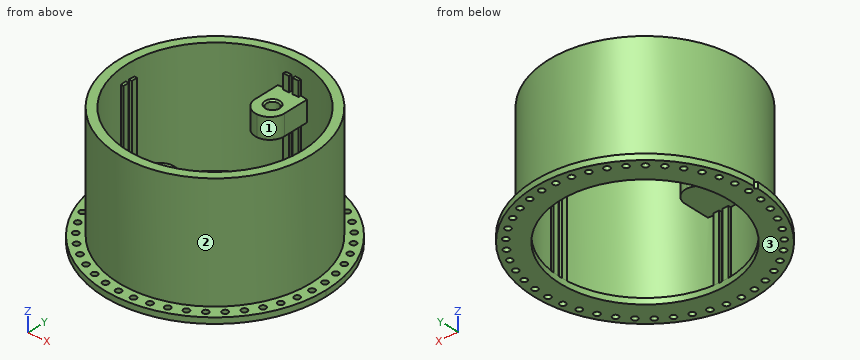
from build123d import *

# Parameters (mm, degrees)
SKETCH_R              = 38
PAD_DEPTH             = 2
SKETCH001_R           = 33
PAD001_DEPTH          = 39.15
SKETCH002_R           = 30
POCKET_DEPTH          = 41.151
SKETCH010_R           = 1
POCKET005_DEPTH       = 5
POLARPATTERN002_COUNT = 45
SKETCH011_R           = 30
PAD005_DEPTH          = 2
SKETCH012_R           = 29
POCKET006_DEPTH       = 2.001
SKETCH013_W           = 2
SKETCH013_H           = 2
PAD006_DEPTH          = 34.15
POLARPATTERN003_COUNT = 4
POCKET008_DEPTH       = 5
SKETCH022_W           = 10
SKETCH022_H           = 15
PAD008_DEPTH          = 7
SKETCH039_R           = 2.05
POCKET025_DEPTH       = 5.5
CHAMFER014_SIZE       = 0.5
FILLET008_R           = 4.99


with BuildPart() as part:
    # Sketch → Pad (new body)
    with BuildSketch(Plane.XY):
        Circle(SKETCH_R)
    extrude(amount=PAD_DEPTH)

    # Sketch001 (on Face3 of Pad) → Pad001 (join)
    with BuildSketch(Plane.XY.offset(2)):
        Circle(SKETCH001_R)
    extrude(amount=PAD001_DEPTH)

    # Sketch002 (on Face5 of Pad001) → Pocket (cut, through all)
    with BuildSketch(Plane.XY.offset(41.15)):
        Circle(SKETCH002_R)
    extrude(amount=-POCKET_DEPTH, mode=Mode.SUBTRACT)

    # Sketch010 (on Face3 of Pocket) → Pocket005 (cut)
    with BuildSketch(Plane.XY.offset(2)):
        with Locations((-35.5, 0)):
            Circle(SKETCH010_R)
    pocket005 = extrude(amount=-POCKET005_DEPTH, mode=Mode.SUBTRACT)

    # PolarPattern002: Pocket005 ×45 about axis
    polarpattern002_axis = Axis((0, 0, 2), (0, 0, 1))
    for i in range(1, POLARPATTERN002_COUNT):
        add(pocket005.rotate(polarpattern002_axis, i * 360 / POLARPATTERN002_COUNT), mode=Mode.SUBTRACT)

    # Sketch011 (on Face2 of PolarPattern002) → Pad005 (join)
    with BuildSketch(Plane(origin=(0, 0, 0), x_dir=(1, 0, 0), z_dir=(0, 0, -1))):
        Circle(SKETCH011_R)
    extrude(amount=-PAD005_DEPTH)

    # Sketch012 (on Face51 of Pad005) → Pocket006 (cut, through all)
    with BuildSketch(Plane.XY.offset(2)):
        Circle(SKETCH012_R)
    extrude(amount=-POCKET006_DEPTH, mode=Mode.SUBTRACT)

    # Sketch013 (on Face51 of Pocket006) → Pad006 (join)
    with BuildSketch(Plane.XY.offset(2)):
        with Locations((-30, 1.6)):
            Rectangle(SKETCH013_W, SKETCH013_H)
        with Locations((-30, -1.6)):
            Rectangle(SKETCH013_W, SKETCH013_H)
    pad006 = extrude(amount=PAD006_DEPTH)

    # PolarPattern003: Pad006 ×4 about axis
    polarpattern003_axis = Axis((0, 0, 2), (0, 0, 1))
    for i in range(1, POLARPATTERN003_COUNT):
        add(pad006.rotate(polarpattern003_axis, i * 360 / POLARPATTERN003_COUNT))

    # Sketch015 → Pocket008 (cut)
    with BuildSketch(Plane.XY.offset(5)):
        Polygon((-38, 0.707107), (-38.707107, 0), (-38, -0.707107), (-37.292893, 0), align=None)
    extrude(amount=-POCKET008_DEPTH, mode=Mode.SUBTRACT)

    # Sketch022 (on DatumPlane) → Pad008 (join)
    with BuildSketch(Plane.XY.offset(24.15)):
        with Locations((0, -23.5)):
            Rectangle(SKETCH022_W, SKETCH022_H)
        with Locations((0, 23.5)):
            Rectangle(SKETCH022_W, SKETCH022_H)
    extrude(amount=PAD008_DEPTH)

    # Sketch039 (on Face85 of Pad008) → Pocket025 (cut)
    with BuildSketch(Plane.XY.offset(31.15)):
        with Locations((0, 22)):
            Circle(SKETCH039_R)
        with Locations((0, -22)):
            Circle(SKETCH039_R)
    extrude(amount=-POCKET025_DEPTH, mode=Mode.SUBTRACT)

    # Chamfer014
    chamfer014_edges = [part.edges().sort_by_distance(p)[0] for p in [
        (-2.05, -22, 31.15),
        (-2.05, 22, 31.15),
    ]]
    chamfer(chamfer014_edges, length=CHAMFER014_SIZE)

    # Fillet008
    fillet008_edges = [part.edges().sort_by_distance(p)[0] for p in [
        (5, -16, 27.65),
        (-5, -16, 27.65),
        (5, 16, 27.65),
        (-5, 16, 27.65),
    ]]
    fillet(fillet008_edges, radius=FILLET008_R)


solid = part.part
The model under review builds one solid part; all positions refer to its coordinate system, in mm. Face numbers are marked on the shaded views. Give positions to 0.01 mm unless a question says otherwise; leave off trailing zeros. Loops run counter-clockwise (first coordinate to the right, second up) from the corner with the lowest first, then second, coordinate; pieces in that order, holes last. Notation, with made-up numbers: (54, 25.5) -> (113, 25.5) arc R13 cw to (113, 34.5) -> close; hole circle Ø9 at (6, 75.5). An arc over 180 degrees is marked (long way). Put each result on its own line as item: value. Start each with the question number.
1. Clearance check with flat-ended pins moving along their axes: P1, Ø3, axis at x = 26.5, z = 17.5, coming from the -Y side; P2, Ø3, axis at y = 5.5, z = 19, coming from the +X side; P3, Ø5, axis at y = -22, z = 12, coming from the -X side; P4, Ø1.8, axis at x = 8.59, y = -34.45, coming from the +Z side. State where each tip first meets the part, or that it passes through.
2. We need section B-B on x = -9. State the section outline as (y, z) points.
3. Mouldability with a two-part tool opening along X and no side actions: class the marked faces 1, 2 and 3 as released by +X, released by -X, zero draft, split by the parting line, or undercut.
4. Wall thickness on probe 1 along Z at (x, y) = (-14.5, -30); probe 2 along Y at (x, z) = (-5, 20); probe 3 along Y at (x, z) = (7.5, 22): over which ranges is each line inside the solid? List them lowest first.
Determined:
1. P1: y = -21.54
1. P2: x = 32.76
1. P3: x = -26.62
1. P4: through
2. outline: (-36.92, 0) -> (-27.57, 0) -> (-27.57, 2) -> (-28.62, 2) -> (-28.62, 41.15) -> (-31.75, 41.15) -> (-31.75, 2) -> (-36.92, 2) -> close; (27.57, 0) -> (36.92, 0) -> (36.92, 2) -> (31.75, 2) -> (31.75, 41.15) -> (28.62, 41.15) -> (28.62, 2) -> (27.57, 2) -> close
3. face 1: undercut
3. face 2: split by the parting line
3. face 3: zero draft
4. probe 1: 0 to 2
4. probe 2: -32.62 to -29.58, 29.58 to 32.62
4. probe 3: -32.14 to -29.05, 29.05 to 32.14
